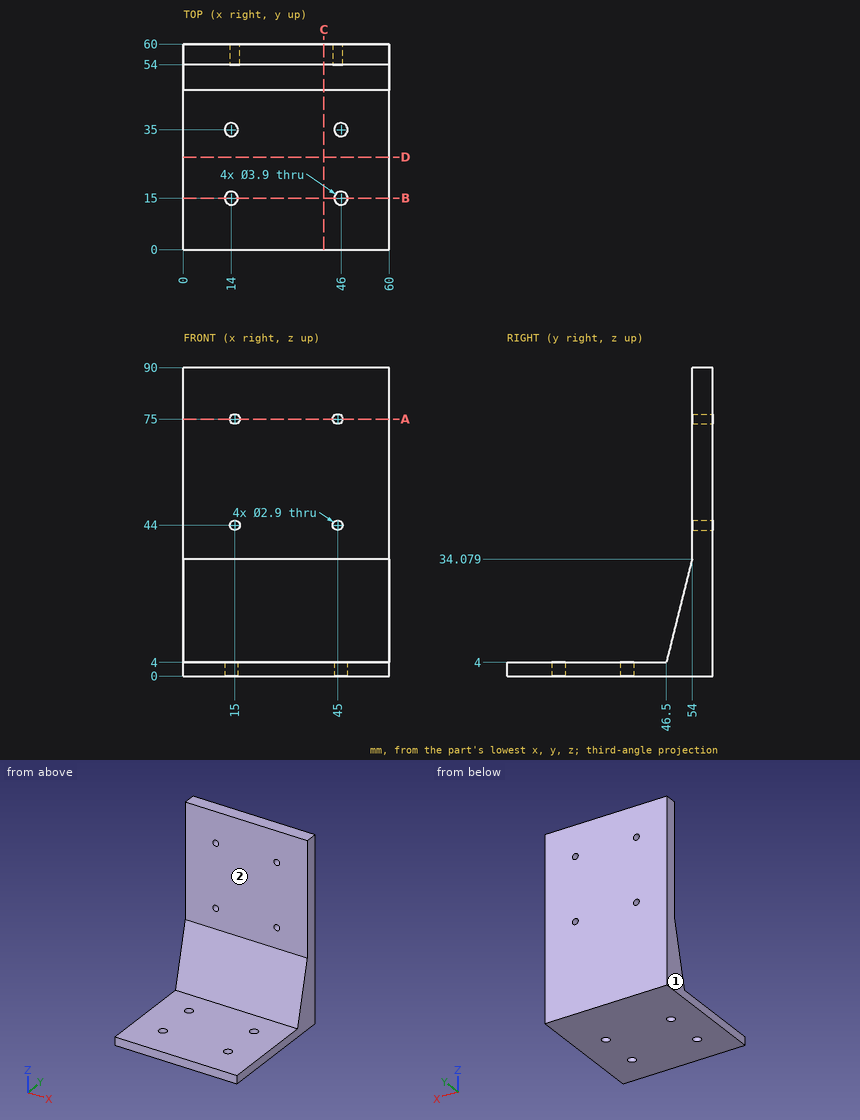
Print and shaded views of the part. All mm, measured from the part's lowest x, y and z. A direction names the side the tool comes from. Round coordinates to 2 decimals unless told otherwise and drop trailing zeros. Write each loop counter-clockwise with the first axis right and the second up, starting at its lowest first coordinate (ties: lowest second). Pieces come first, ordered by that corner, then holes. Notation, with made-up numbers: M 31,-36 L 49,-36 A20 ccw 49,-6 Z; hole C 26,-37.75 d2. An arc over 180 degrees is marked long. Use a Markdown table: item, result. Add a question column.
1. Flat gauge pins, fed straight in: P1, Ø3, axis at x = 10, z = 24, coming from the -Y side; P2, Ø14, axis at x = 30, y = 29, coming from the +Z side; P3, Ø1.5, axis at x = 52, z = 37, coming from the -Y side; P4, Ø2.5, axis at x = 46, y = 35, coming from the -Z side. Where does each tip first touch, or does it go through?
2. 3-axis set-ups, long thin cutter, end or side, ignore diameter. For the marked faces 1 and 2: which of +Z, -Z, +X, -X, +Y, -Y reach the whole face in a straight line?
3. Slice it at A-A on z = 75. Give the cut face in (x, y), then the cut area to 3 significant figures.
4. Drill centre lines: probe 1 along X at (y, z) = (56.15, 75); probe 2 along Z at (x, y) = (15, 55); probe 3 along Y at (x, z) = (46, 1.1). Where is each one in solid material? Low to high.
5. Slice it at B-B on y = 15. Give the cut face in (x, z).
6. Slice it at C-C on x = 41. Give the cut face in (y, z).
7. Slice it at D-D on y = 27. Give the cut face in (x, z).
Reply:
| question | item | result |
|---|---|---|
| 1 | P1 | stops at y = 51.11 |
| 1 | P2 | stops at z = 4 |
| 1 | P3 | stops at y = 54 |
| 1 | P4 | passes through |
| 2 | face 1 | +Z, -Z, -X, +Y, -Y |
| 2 | face 2 | +Z, +X, -X, -Y |
| 3 | outline | M 0,54 L 13.55,54 L 13.55,60 L 0,60 Z; M 16.45,54 L 43.55,54 L 43.55,60 L 16.45,60 Z; M 46.45,54 L 60,54 L 60,60 L 46.45,60 Z |
| 3 | area | 325 mm^2 |
| 4 | probe 1 | x = 0 to 13.55, 16.45 to 43.55, 46.45 to 60 |
| 4 | probe 2 | z = 0 to 42.55, 45.45 to 73.55, 76.45 to 90 |
| 4 | probe 3 | y = 0 to 13.05, 16.95 to 33.05, 36.95 to 60 |
| 5 | outline | M 0,0 L 12.05,0 L 12.05,4 L 0,4 Z; M 15.95,0 L 44.05,0 L 44.05,4 L 15.95,4 Z; M 47.95,0 L 60,0 L 60,4 L 47.95,4 Z |
| 6 | outline | M 0,0 L 60,0 L 60,90 L 54,90 L 54,34.08 L 46.5,4 L 0,4 Z |
| 7 | outline | M 0,0 L 60,0 L 60,4 L 0,4 Z |
